from build123d import *

# Parameters (mm, degrees)
SKETCH1_R           = 1
SKETCH1_R_2         = 2
SKETCH1_R_3         = 1.5
BOSS_EXTRUDE1_DEPTH = 5
SKETCH3_R           = 1
BOSS_EXTRUDE2_DEPTH = 10
CUT_EXTRUDE1_DEPTH  = 1.5


with BuildPart() as part:
    # Sketch1 → Boss-Extrude1 (new body)
    with BuildSketch(Plane.XY):
        with BuildLine():
            Line((-16, 0), (-16, 80))
            Line((-16, 80), (16, 80))
            Line((16, 80), (16, 0))
            ThreePointArc((16, 0), (0, -16), (-16, 0))
        make_face()
        with Locations((0, -8)):
            Circle(SKETCH1_R, mode=Mode.SUBTRACT)
        Circle(SKETCH1_R_2, mode=Mode.SUBTRACT)
        with Locations((-8, 0)):
            Circle(SKETCH1_R, mode=Mode.SUBTRACT)
        with Locations((0, 8)):
            Circle(SKETCH1_R, mode=Mode.SUBTRACT)
        with Locations((8, 0)):
            Circle(SKETCH1_R, mode=Mode.SUBTRACT)
        with Locations((11, 75)):
            Circle(SKETCH1_R_3, mode=Mode.SUBTRACT)
        with Locations((-11, 75)):
            Circle(SKETCH1_R_3, mode=Mode.SUBTRACT)
        with Locations((-11, 30)):
            Circle(SKETCH1_R_3, mode=Mode.SUBTRACT)
        with Locations((11, 30)):
            Circle(SKETCH1_R_3, mode=Mode.SUBTRACT)
    extrude(amount=BOSS_EXTRUDE1_DEPTH)

    # Sketch3 → Boss-Extrude2 (add)
    with BuildSketch(Plane.XY):
        Polygon((-16, 80), (16, 80), (16, 100), (11, 100), (11, 86), (-11, 86), (-11, 100), (-16, 100), align=None)
        with Locations((-13.5, 95.8)):
            Circle(SKETCH3_R, mode=Mode.SUBTRACT)
        with Locations((13.5, 95.8)):
            Circle(SKETCH3_R, mode=Mode.SUBTRACT)
        with Locations((13.5, 87.8)):
            Circle(SKETCH3_R, mode=Mode.SUBTRACT)
        with Locations((-13.5, 87.8)):
            Circle(SKETCH3_R, mode=Mode.SUBTRACT)
    extrude(amount=BOSS_EXTRUDE2_DEPTH)

    # Sketch5 → Cut-Extrude1 (cut)
    with BuildSketch(Plane.XY.offset(5)):
        Polygon((-8.113248654, 75), (-9.556624327, 77.5), (-12.443375673, 77.5), (-13.886751346, 75), (-12.443375673, 72.5), (-9.556624327, 72.5), align=None)
        Polygon((-8.113248654, 30), (-9.556624327, 32.5), (-12.443375673, 32.5), (-13.886751346, 30), (-12.443375673, 27.5), (-9.556624327, 27.5), align=None)
        Polygon((13.886751346, 30), (12.443375673, 32.5), (9.556624327, 32.5), (8.113248654, 30), (9.556624327, 27.5), (12.443375673, 27.5), align=None)
        Polygon((13.886751346, 75), (12.443375673, 77.5), (9.556624327, 77.5), (8.113248654, 75), (9.556624327, 72.5), (12.443375673, 72.5), align=None)
    extrude(amount=-CUT_EXTRUDE1_DEPTH, mode=Mode.SUBTRACT)


solid = part.part
Work out the finished part from the listing and answer in its coordinate system (mm). A direction names the side the tool comes from. Give positions to 0.01 mm unless a question says otherwise; leave off trailing zeros. Write each loop counter-clockwise with the first axis right and the second up, starting at its lowest first coordinate (ties: lowest second). Pieces come first, ordered by that corner, then holes. Notation, with made-up numbers: (26.25, 54) - (39.25, 54) arc R12 cw to (39.25, 66) - close; hole circle Ø10 at (12, 9). An arc over 180 degrees is marked (long way). One line per item, written item: value. Start each with the question number.
1. Consider probe 1 along Y at (x, z) = (-13.5, 7); probe 2 along X at (y, z) = (88, 4); probe 3 along Y at (x, z) = (0, 1.1). Determine where each line is inside the solid, lowest interval first.
2. For a pull along Y with two mould halves and no side action, classify faces 6 (the flat face through (14, 100, 5)), 7 (the cylindrical face through (13.37, 96.79, 4.93)), 8 (the flat face through (-0.2, 85.7, 10)) as +Y half, -Y half, draft (parallel to the pull), parting line (faces both ways), or undercut.
3. For faces 1 (the flat face through (-11, 93, 5)), 2 (the flat face through (0, 43, 0)), 3 (the flat face through (-9.76, 31.15, 3.5)), 4 (the cylindrical face through (-8.8, -0.6, 2.5)), 5 (the flat face through (0, 80, 7)), determine the directions among +Z, -Z, +X, -X, +Y, -Y from which every point of the face is accessible in a straight line to the end or side of a thin tool.
4. Find section A-A (y = 8). Write down the section's boundary in (x, z).
5. Find section B-B (x = 0). Write down the section's boundary in (y, z).
6. Find section D-D (z = 2.25). State how many separate pieces and enclosed holes the cut face has, then the cut area to 3 significant figures.
7. Find section C-C (y = 87.8). Write down the section's boundary in (x, z), then the cut area to 3 significant figures.
8. Given pin 1 (0.8 mm diameter, centred on x = -10.5, z = 4.5, fed in from -Y); pin 2 (3 mm diameter, centred on x = 0, y = -8, fed in from +Z); pin 3 (5 mm diameter, centred on x = 1, z = 5, fed in from +Y), each flat-ended and moving along its own axis, determine where each tip first touches the part or whether it passes through.
Geometry results:
1. probe 1: 80 to 86.8, 88.8 to 94.8, 96.8 to 100
1. probe 2: -16 to -14.48, -12.52 to -11, 11 to 12.52, 14.48 to 16
1. probe 3: -16 to -9, -7 to -2, 2 to 7, 9 to 86
2. face 6: +Y half
2. face 7: undercut
2. face 8: draft
3. face 1: +Z, -Z, +Y
3. face 2: -Z, +X, -X, +Y, -Y
3. face 3: +Z
3. face 4: +Z, -Z
3. face 5: +Z, +X, -X, -Y
4. outline: (-16, 0) - (-1, 0) - (-1, 5) - (-16, 5) - close; (1, 0) - (16, 0) - (16, 5) - (1, 5) - close
5. outline: (-16, 0) - (-9, 0) - (-9, 5) - (-16, 5) - close; (-7, 0) - (-2, 0) - (-2, 5) - (-7, 5) - close; (2, 0) - (7, 0) - (7, 5) - (2, 5) - close; (9, 0) - (86, 0) - (86, 10) - (80, 10) - (80, 5) - (9, 5) - close
6. separate pieces: 1
6. enclosed holes: 13
6. area: 3,230 mm2
7. outline: (-16, 0) - (-14.5, 0) - (-14.5, 10) - (-16, 10) - close; (-12.5, 0) - (-11, 0) - (-11, 10) - (-12.5, 10) - close; (11, 0) - (12.5, 0) - (12.5, 10) - (11, 10) - close; (14.5, 0) - (16, 0) - (16, 10) - (14.5, 10) - close
7. area: 60.0 mm2
8. pin 1: y = -12.41
8. pin 2: z = 5
8. pin 3: y = 86
